Could you check a few things on this model? Use its own coordinates, in mm. A direction names the side the tool comes from. Give positions to 0.01 mm unless a question says otherwise; leave off trailing zeros. Loops run counter-clockwise (first coordinate to the right, second up) from the corner with the lowest first, then second, coordinate; pieces in that order, holes last. Notation, with made-up numbers: M 24.25,36.5 L 74.25,36.5 A9 cw 74.25,47.5 Z; hole C 70.5,-29.5 d3. An arc over 180 degrees is marked long. Return JSON: item names as keys, results as strings. Group by question number.
1. If we section it at B-B (z = -175.5): Write out the boundary of the cut face in (x, y), plus the area to 3 significant figures.
2. Please list where these lines run through material, in increasing order: line 1 (Z direction, x = -6, y = 16.5); line 2 (Z direction, x = -3.5, y = 9.5); line 3 (Z direction, x = -11.25, y = 18).
3. If we mould it in two halves opening along X, with no side actions, what happens to faces 5 (the cylindrical face through (-4.66, 19.19, -20.11)), 6 (the flat face through (-8, 20, -127)), 7 (the flat face through (-14, 10, -111))? For each: +X half, -X half, draft (parallel to the pull), parting line (faces both ways), or undercut.
4. If we section it at A-A (y = 10): Write out the boundary of the cut face in (x, z), plus the area to 3 significant figures.
5. For faces 1 (the flat face through (-12.45, 1.52, -138.46)), 2 (the flat face through (-13, 10, -18)), 3 (the flat face through (-14, 10, -32)), 4 (the cylindrical face through (-6.33, 19.19, -234.48)), which set-ups out of +Z, -Z, +X, -X, +Y, -Y let a thin tool reach every point of the face, with its end or its side?
6. For pin 1 (6 mm diameter, centred on y = 16.5, z = -109, fed in from -X); pin 2 (11 mm diameter, centred on y = 12.5, z = -185.5, fed in from -X); pin 3 (2 mm diameter, centred on x = -13.5, y = 8.5, fed in from -Z), each with a flat end and sliding along its axis, tell me the tip position at first contact or that it passes through.
```python
from build123d import *

# Parameters (mm, degrees)
BOSS_EXTRUDE1_DEPTH                          = 20
SKETCH2_R                                    = 4.3
CUT_EXTRUDE1_DEPTH                           = 13
CBORE_START                                  = 18.4
CBORE_FOR_M2_PAN_HEAD_MACHINE_SCREW1_OUT_R   = 2.5
CBORE_FOR_M2_PAN_HEAD_MACHINE_SCREW1_DEPTH   = 1.6
CBORE_START_2                                = 14.156921837
CBORE_FOR_M2_PAN_HEAD_MACHINE_SCREW1_2_O_R   = 1.1
CBORE_FOR_M2_PAN_HEAD_MACHINE_SCREW1_2_DEPTH = 4.243078163
CHAMFER1_SIZE                                = 3
CHAMFER2_SIZE                                = 0.8
SKETCH2_5_R                                  = 4.3
CUT_EXTRUDE5_DEPTH                           = 252.443830706


# Read off the part's stored shape, not the designer's step: CBORE for M2 Pan Head Machine Screw1
with BuildPart() as part:
    # Sketch1 → Boss-Extrude1 (new body)
    with BuildSketch(Plane(origin=(0, 0, 0), x_dir=(1, 0, 0), z_dir=(0, 1, 0))):
        Polygon((-10, 214), (-10, 143), (-18, 135), (-18, 115), (-10, 107), (-10, 36), (-18, 28), (-18, 8), (-10, 0), (0, 0), (0, 250), (-10, 250), (-18, 242), (-18, 222), align=None)
    extrude(amount=BOSS_EXTRUDE1_DEPTH)

    # Sketch2 → Cut-Extrude1 (cut)
    with BuildSketch(Plane(origin=(0, 0, 0), x_dir=(0, 0, -1), z_dir=(1, 0, 0))):
        with Locations((18, 10)):
            Circle(SKETCH2_R)
        with Locations((125, 10)):
            Circle(SKETCH2_R)
        with Locations((232, 10)):
            Circle(SKETCH2_R)
    extrude(amount=-CUT_EXTRUDE1_DEPTH, mode=Mode.SUBTRACT)

    # CBORE for M2 Pan Head Machine Screw1 out → CBORE for M2 Pan Head Machine Screw1 (cut)
    with BuildSketch(Plane(origin=(0, 0, 0), x_dir=(1, 0, 0), z_dir=(0, 1, 0)).offset(CBORE_START)):
        with Locations((-6, 18)):
            Circle(CBORE_FOR_M2_PAN_HEAD_MACHINE_SCREW1_OUT_R)
        with Locations((-6, 232)):
            Circle(CBORE_FOR_M2_PAN_HEAD_MACHINE_SCREW1_OUT_R)
        with Locations((-6, 125)):
            Circle(CBORE_FOR_M2_PAN_HEAD_MACHINE_SCREW1_OUT_R)
    extrude(amount=CBORE_FOR_M2_PAN_HEAD_MACHINE_SCREW1_DEPTH, mode=Mode.SUBTRACT)

    # CBORE for M2 Pan Head Machine Screw1 2 o → CBORE for M2 Pan Head Machine Screw1 2 (cut)
    with BuildSketch(Plane(origin=(0, 0, 0), x_dir=(1, 0, 0), z_dir=(0, 1, 0)).offset(CBORE_START_2)):
        with Locations((-6, 18)):
            Circle(CBORE_FOR_M2_PAN_HEAD_MACHINE_SCREW1_2_O_R)
        with Locations((-6, 232)):
            Circle(CBORE_FOR_M2_PAN_HEAD_MACHINE_SCREW1_2_O_R)
        with Locations((-6, 125)):
            Circle(CBORE_FOR_M2_PAN_HEAD_MACHINE_SCREW1_2_O_R)
    extrude(amount=CBORE_FOR_M2_PAN_HEAD_MACHINE_SCREW1_2_DEPTH, mode=Mode.SUBTRACT)

    # Chamfer1
    chamfer1_edges = [part.edges().sort_by_distance(p)[0] for p in [
        (-14, 20, -246),
        (-5, 0, 0),
        (-14, 0, -4),
        (-18, 0, -18),
        (-14, 0, -32),
        (-10, 0, -71.5),
        (-14, 0, -111),
        (-18, 0, -125),
        (-14, 0, -139),
        (-18, 20, -232),
        (-10, 0, -178.5),
        (-14, 0, -218),
        (-18, 0, -232),
        (-14, 0, -246),
        (-5, 0, -250),
        (-14, 20, -218),
        (-10, 20, -178.5),
        (-14, 20, -139),
        (-18, 20, -125),
        (-14, 20, -111),
        (-10, 20, -71.5),
        (-14, 20, -32),
        (-18, 20, -18),
        (-14, 20, -4),
        (-5, 20, 0),
        (-5, 20, -250),
    ]]
    chamfer(chamfer1_edges, length=CHAMFER1_SIZE)

    # Chamfer2
    chamfer2_edges = [part.edges().sort_by_distance(p)[0] for p in [
        (0, 10, 0),
        (0, 0, -125),
        (0, 10, -250),
        (0, 20, -125),
        (0, 18.5, -1.5),
        (0, 18.5, -248.5),
        (0, 1.5, -248.5),
        (0, 1.5, -1.5),
    ]]
    chamfer(chamfer2_edges, length=CHAMFER2_SIZE)

    # Sketch2<5> → Cut-Extrude5 (cut, through all)
    with BuildSketch(Plane(origin=(0, 0, 0), x_dir=(0, 0, -1), z_dir=(1, 0, 0))):
        with Locations((232, 10)):
            Circle(SKETCH2_5_R)
    extrude(amount=-CUT_EXTRUDE5_DEPTH, mode=Mode.SUBTRACT)


solid = part.part
```
Answer:
{
 "1": {"outline": "M -10,3 L -7,0 L -0.8,0 L 0,0.8 L 0,19.2 L -0.8,20 L -7,20 L -10,17 Z", "area": "190 mm²"},
 "2": {"line 1": "z = -250 to -233.1, -230.9 to -126.1, -123.9 to -19.1, -16.9 to 0", "line 2": "z = -250 to -236.27, -227.73 to -129.27, -120.73 to -22.27, -13.73 to 0", "line 3": "z = -247.34 to -216.66, -140.34 to -109.66, -33.34 to -2.66"},
 "3": {"face 5": "undercut", "face 6": "draft", "face 7": "-X half"},
 "4": {"outline": "M -18,-242 L -10,-250 L -0.8,-250 L 0,-249.2 L 0,-236.3 L -18,-236.3 Z; M -18,-227.7 L 0,-227.7 L 0,-129.3 L -13,-129.3 L -13,-120.7 L 0,-120.7 L 0,-22.3 L -13,-22.3 L -13,-13.7 L 0,-13.7 L 0,-0.8 L -0.8,0 L -10,0 L -18,-8 L -18,-28 L -10,-36 L -10,-107 L -18,-115 L -18,-135 L -10,-143 L -10,-214 L -18,-222 Z", "area": "2,790 mm²"},
 "5": {"face 1": "-X, -Y", "face 2": "+X", "face 3": "-X, +Y, -Y", "face 4": "+Y"},
 "6": {"pin 1": "stops at x = -15", "pin 2": "stops at x = -10", "pin 3": "stops at z = -247.5"}
}
